Here's the drawing with two shaded views (mm, measured from the low corner). I have some questions. A direction names the side the tool comes from. Round coordinates to 2 decimals unless told otherwise and drop trailing zeros. Write each loop counter-clockwise with the first axis right and the second up, starting at its lowest first coordinate (ties: lowest second). Pieces come first, ordered by that corner, then holes. Notation, with made-up numbers: M 89.5,33 L 124.5,33 A23 cw 124.5,70 Z; hole C -17,-11.75 d10. An arc over 180 degrees is marked long. Answer as a JSON object with one key per item and string values. Group by question number.
1) Suppose I cut it at C-C, the plane y = 10.25. Write out the boundary of the cut face in (x, z), and give its area (4 significant figures).
2) On a 3-axis mill with a long thin cutter (end or side, diameter ignored), from which of +Z, -Z, +X, -X, +Y, -Y can I reach the whole of each face in a straight line? I mean the marked faces 1, 2 and 3. Say none if no direction works.
3) Suppose I cut it at B-B, the plane z = 3.75. Write out the boundary of the cut face in (x, y), and give its area (3 significant figures).
4) Please list where these lines run through material, in increasing order: L1, parallel to X at y = 5, z = 1.5; L2, parallel to X at y = 20.75, z = 7.25; L3, parallel to Y at x = 9.5, z = 4. Write a range as [from, to].
5) Suppose I cut it at A-A, the plane x = 28.5. Write out the boundary of the cut face in (y, z).
6) I'm going to push flat-ended pins straight in: pin 1 Ø4 at (y, z) = (18.5, 2.5) entering from +X; pin 2 Ø6 at (x, z) = (7.5, 2) entering from -Y; pin 3 Ø2.5 at (y, z) = (13.5, 7) entering from +X; pin 4 Ø0.6 at (x, z) = (23, 6.5) entering from -Y. Where does each tip first touch, or does it pass through?
7) Suppose I cut it at D-D, the plane x = 3. Write out the boundary of the cut face in (y, z), and give its area (4 significant figures).
8) If we mould it in two halves opening along Y, with no side actions, what happens to the marked faces 4, 5, 6 and 7? For each: +Y half, -Y half, draft (parallel to the pull), parting line (faces both ways), or undercut.
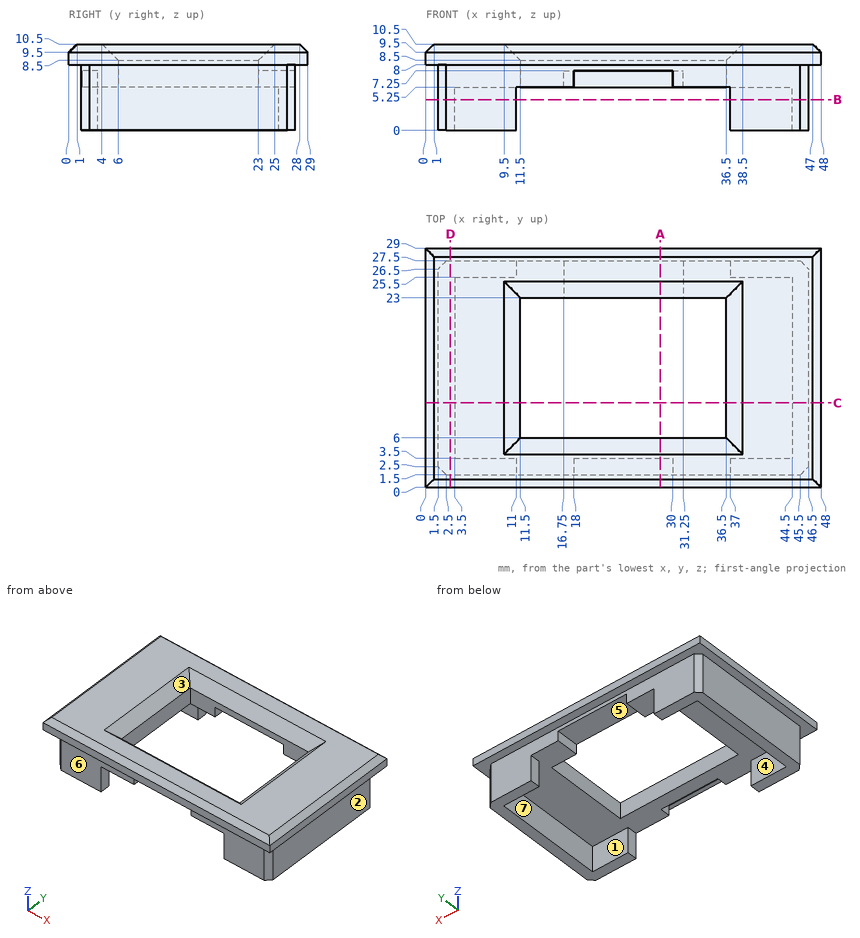
Results:
{
 "1": {"outline": "M 0,8 L 1.5,8 L 1.5,0 L 3.5,0 L 3.5,5.25 L 11.5,5.25 L 11.5,8.5 L 9.5,10.5 L 1,10.5 L 0,9.5 Z; M 36.5,5.25 L 44.5,5.25 L 44.5,0 L 46.5,0 L 46.5,8 L 48,8 L 48,9.5 L 47,10.5 L 38.5,10.5 L 36.5,8.5 Z", "area": "128.5 mm^2"},
 "2": {"face 1": "-Z", "face 2": "-Z, +X, +Y, -Y", "face 3": "+Z"},
 "3": {"outline": "M 1.5,2.5 L 2.5,1.5 L 11,1.5 L 11,3.5 L 3.5,3.5 L 3.5,25.5 L 11,25.5 L 11,27.5 L 2.5,27.5 L 1.5,26.5 Z; M 37,1.5 L 45.5,1.5 L 46.5,2.5 L 46.5,26.5 L 45.5,27.5 L 37,27.5 L 37,25.5 L 44.5,25.5 L 44.5,3.5 L 37,3.5 Z", "area": "162 mm^2"},
 "4": {"L1": "[1.5, 3.5], [44.5, 46.5]", "L2": "[1.5, 11.5], [36.5, 46.5]", "L3": "[1.5, 3.5], [25.5, 27.5]"},
 "5": {"outline": "M 0,8 L 1.5,8 L 1.5,7.25 L 3.5,7.25 L 3.5,5.25 L 6,5.25 L 6,8.5 L 4,10.5 L 1,10.5 L 0,9.5 Z; M 23,7.25 L 27.5,7.25 L 27.5,8 L 29,8 L 29,9.5 L 28,10.5 L 25,10.5 L 23,8.5 Z"},
 "6": {"pin 1": "x = 46.5", "pin 2": "y = 1.5", "pin 3": "x = 48", "pin 4": "y = 3.5"},
 "7": {"outline": "M 0,8 L 1.5,8 L 1.5,0 L 27.5,0 L 27.5,8 L 29,8 L 29,9.5 L 28,10.5 L 1,10.5 L 0,9.5 Z", "area": "279.5 mm^2"},
 "8": {"face 4": "undercut", "face 5": "draft", "face 6": "-Y half", "face 7": "undercut"}
}
